Print and shaded views of the part. All mm, measured from the part's lowest x, y and z. A direction names the side the tool comes from. Round coordinates to 2 decimals unless told otherwise and drop trailing zeros. Use one line per item in the form item = value.
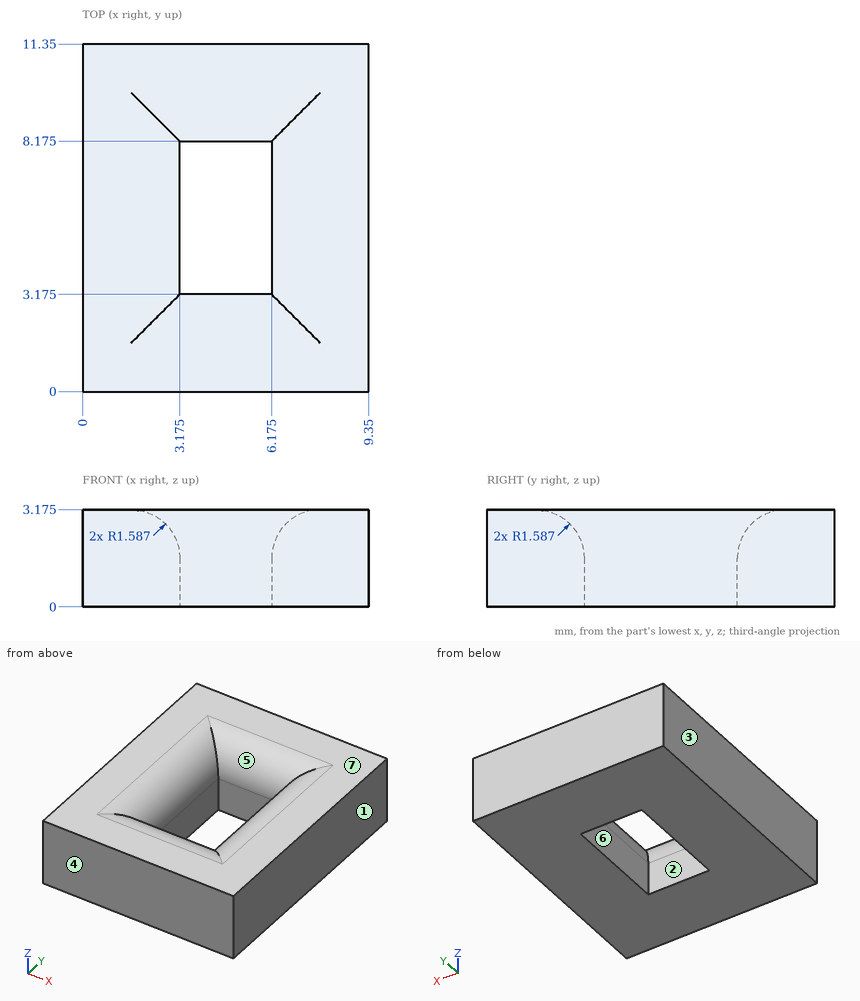
1) Drill centre lines: probe 1 along X at (y, z) = (7, 2.9); probe 2 along Y at (x, z) = (5.5, 2.2); probe 3 along Y at (x, z) = (6.75, 2.85). Where is each one in solid material? Low to high.
Report:
probe_1 = 0 to 2.48, 6.87 to 9.35
probe_2 = 0 to 3.05, 8.3 to 11.35
probe_3 = 0 to 2.55, 8.8 to 11.35
2) Two-plate mould, pull along X, no slides. Class the marked faces 1, 2, 3 and 4: +X half, -X half, draft (parallel to the pull), parting line (faces both ways), or undercut.
Report:
face_1 = +X half
face_2 = undercut
face_3 = -X half
face_4 = draft
3) Tool access for the marked faces 5, 6 and 7: list every direction of +Z, -Z, +X, -X, +Y, -Y with a clear straight run to the whole face (end or side of a thin tool).
Report:
face_5 = +Z
face_6 = +Z, -Z
face_7 = +Z, +X, -X, +Y, -Y
